Design review of the part built by this model. Coordinates are the model's own, in mm. A direction names the side the tool comes from. Coordinates: 2 decimals unless noted, no trailing zeros. Write each loop counter-clockwise with the first axis right and the second up, starting at its lowest first coordinate (ties: lowest second). Pieces come first, ordered by that corner, then holes.
Q1. For faces 4 (the flat face through (-21, -33.272, 48)), 5 (the flat face through (-19.834, -48, 48)), 6 (the flat face through (-22.834, -47, 50)), list the 3-axis set-ups (+Z, -Z, +X, -X, +Y, -Y) from which the entire face can be reached by the end or side of a thin tool; tool diameter is ignored.
Q2. Take a section at D-D, the plane y = -50. Write out the cut boundary in (x, z), plus the area to 3 significant figures.
Q3. Take a section at B-B, the plane z = 91.5. Write out the cut boundary in (x, y), plus the area to 3 significant figures.
Q4. Take a section at A-A, the plane y = -8.5. Write out the cut boundary in (x, z), plus the area to 3 significant figures.
Q5. The part is to be moulded in two halves that separate along X. For faces 1 (the flat face through (53, -63.272, 50)), 2 (the flat face through (54.166, -47, 50)), 3 (the flat face through (15, -33, 98)), say which applies: released by +X, released by -X, zero draft, split by the parting line, or undercut.
Q6. Take a section at C-C, the plane x = -13.5. Write out the cut boundary in (y, z).
Q7. For pin 1 Ø2.5 at (x, z) = (53, 67) entering from +Y; pin 2 Ø23 at (x, y) = (5, -31.5) entering from -Z; pin 3 Ø0.6 at (x, z) = (7.5, 99) entering from +Y, all flat-tipped, find the tip position at first contact; note any pin that passes through.
Q8. For L1, parallel to X at y = -45.5, z = 45; L2, parallel to Z at x = -4.5, y = -45.5, list the stretches that pass through material, from the lowest coordinate up.
from build123d import *

# Parameters (mm, degrees)
SKETCH_1_W          = 77
SKETCH_1_H          = 80
EXTRUDE_1_DEPTH     = 100
SKETCH_2_W          = 45
SKETCH_2_H          = 35
CUT_EXTRUDE_1_DEPTH = 100
SKETCH_3_W          = 71
SKETCH_3_H          = 80
CUT_EXTRUDE_2_DEPTH = 98
SKETCH_5_W          = 98
SKETCH_5_H          = 50
CUT_EXTRUDE_3_DEPTH = 98


with BuildPart() as part:
    # 草图1 → 凸台-拉伸1 (new body)
    with BuildSketch(Plane.XY):
        with Locations((15.665517241, -23.272413793)):
            Rectangle(SKETCH_1_W, SKETCH_1_H)
    extrude(amount=EXTRUDE_1_DEPTH)

    # 草图2 → 切除-拉伸1 (cut)
    with BuildSketch(Plane.XY.offset(100)):
        with Locations((15.665517241, -0.772413793)):
            Rectangle(SKETCH_2_W, SKETCH_2_H)
    extrude(amount=-CUT_EXTRUDE_1_DEPTH, mode=Mode.SUBTRACT)

    # 草图3 → 切除-拉伸2 (cut)
    with BuildSketch(Plane(origin=(0, 0, 0), x_dir=(-1, 0, 0), z_dir=(0, 0, -1))):
        with Locations((-15.665517241, -23.272413793)):
            Rectangle(SKETCH_3_W, SKETCH_3_H)
    extrude(amount=-CUT_EXTRUDE_2_DEPTH, mode=Mode.SUBTRACT)

    # 草图5 → 切除-拉伸3 (cut)
    with BuildSketch(Plane.ZY.offset(22.834482759)):
        with Locations((49, -8.272413793)):
            Rectangle(SKETCH_5_W, SKETCH_5_H)
    extrude(amount=-CUT_EXTRUDE_3_DEPTH, mode=Mode.SUBTRACT)


solid = part.part
Responses:
1. face 4: -Z, +X, -X, +Y
1. face 5: -Z, +Y, -Y
1. face 6: +Z, -Z, -X, +Y, -Y
2. outline: (-22.83, 0) - (-19.83, 0) - (-19.83, 98) - (51.17, 98) - (51.17, 0) - (54.17, 0) - (54.17, 100) - (-22.83, 100) - close
2. area: 742 mm2
3. outline: (-22.83, -63.27) - (-19.83, -63.27) - (-19.83, -33.27) - (-22.83, -33.27) - close; (51.17, -63.27) - (54.17, -63.27) - (54.17, -33.27) - (51.17, -33.27) - close
3. area: 180 mm2
4. outline: (-22.83, 98) - (-6.83, 98) - (-6.83, 100) - (-22.83, 100) - close; (38.17, 98) - (54.17, 98) - (54.17, 100) - (38.17, 100) - close
4. area: 64.0 mm2
5. face 1: zero draft
5. face 2: released by +X
5. face 3: undercut
6. outline: (-63.27, 98) - (16.73, 98) - (16.73, 100) - (-63.27, 100) - close
7. pin 1: stops at y = -33.27
7. pin 2: stops at z = 98
7. pin 3: stops at y = -18.27
8. L1: x = -22.83 to -19.83, 51.17 to 54.17
8. L2: z = 98 to 100
